The model under review builds one solid part; all positions refer to its coordinate system, in mm. Face numbers are marked on the shaded views. Coordinates: 2 decimals unless noted, no trailing zeros. Order: outer loops, then holes, each group sorted by start corner. A loop starts at its lowest first (then second) coordinate and runs counter-clockwise, first axis right, second up. Notation, with made-up numbers: M 8,-3 L 28,-3 A28 ccw 28,31 Z; hole C 29,-23.5 d9. An arc over 180 degrees is marked long. Write each question's results on one line, items separated by ' | '.
from build123d import *

# Parameters (mm, degrees)
SKETCH_R     = 2.5
SKETCH_R_2   = 1.6
PAD_DEPTH    = 3
SKETCH001_W  = 6.4
SKETCH001_H  = 103.817123
POCKET_DEPTH = 1


with BuildPart() as part:
    # Sketch → Pad (new body)
    with BuildSketch(Plane.XY):
        Polygon((0, 0), (38.400002, 0), (38.4, 61), (0, 61), align=None)
        with Locations((10, 46)):
            Circle(SKETCH_R, mode=Mode.SUBTRACT)
        with Locations((10, 26)):
            Circle(SKETCH_R, mode=Mode.SUBTRACT)
        with Locations((10, 6)):
            Circle(SKETCH_R, mode=Mode.SUBTRACT)
        with Locations((21.5, 54)):
            Circle(SKETCH_R_2, mode=Mode.SUBTRACT)
        with Locations((21.5, 7)):
            Circle(SKETCH_R_2, mode=Mode.SUBTRACT)
        with Locations((34.900002, 7)):
            Circle(SKETCH_R_2, mode=Mode.SUBTRACT)
        with Locations((34.900002, 54)):
            Circle(SKETCH_R_2, mode=Mode.SUBTRACT)
        with Locations((34.900002, 30.5)):
            Circle(SKETCH_R_2, mode=Mode.SUBTRACT)
        with Locations((21.5, 30.5)):
            Circle(SKETCH_R_2, mode=Mode.SUBTRACT)
    extrude(amount=PAD_DEPTH)

    # Sketch001 (on Face15 of Pad) → Pocket (cut)
    with BuildSketch(Plane.XY.offset(3)):
        with Locations((28.2, 19.77481)):
            Rectangle(SKETCH001_W, SKETCH001_H)
    extrude(amount=-POCKET_DEPTH, mode=Mode.SUBTRACT)


solid = part.part
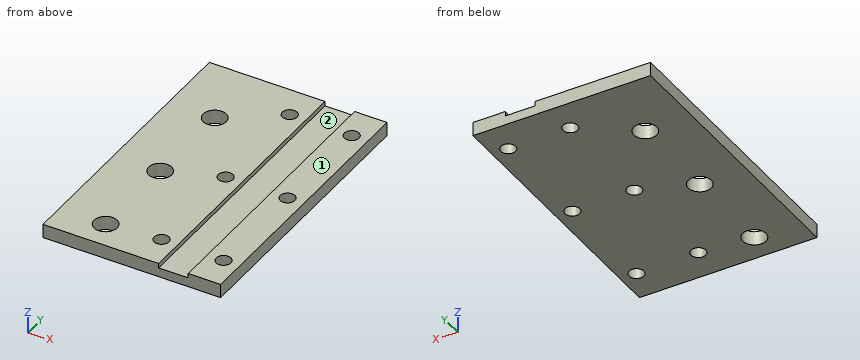
1) Take a section at C-C on z = 0.55. Count the separate pieces of the cut face and the enclosed holes in it, plus the area to 3 significant figures.
Solutions:
separate pieces: 1 | enclosed holes: 9 | area: 2,240 mm2
2) To check wall thickness, follow line 1 along Y through (x, z) = (21.5, 1.65); line 2 along Y through (x, z) = (10, 1.45); line 3 along X through (y, z) = (15, 2.25). State the ranges of each line that lie inside material, in increasing order.
Solutions:
line 1: 0 to 5.4, 8.6 to 28.9, 32.1 to 52.4, 55.6 to 61 | line 2: 0 to 3.5, 8.5 to 23.5, 28.5 to 43.5, 48.5 to 61 | line 3: 0 to 25, 31.4 to 38.4
3) For pin 1 (2 mm diameter, centred on x = 29, y = 27, fed in from +Z); pin 2 (4 mm diameter, centred on x = 10, y = 26, fed in from +Z); pin 3 (4 mm diameter, centred on x = 34.9, y = 54, fed in from +Z), all flat-tipped, find the tip position at first contact; note any pin that passes through.
Solutions:
pin 1: z = 2 | pin 2: through | pin 3: z = 3
4) Take a section at D-D on y = 19. State the section outline as (x, z) points.
Solutions:
outline: M 0,0 L 38.4,0 L 38.4,3 L 31.4,3 L 31.4,2 L 25,2 L 25,3 L 0,3 Z
5) Take a section at B-B on y = 30.5. State the section outline as (x, z) points.
Solutions:
outline: M 0,0 L 19.9,0 L 19.9,3 L 0,3 Z; M 23.1,0 L 33.3,0 L 33.3,3 L 31.4,3 L 31.4,2 L 25,2 L 25,3 L 23.1,3 Z; M 36.5,0 L 38.4,0 L 38.4,3 L 36.5,3 Z
6) The part is to be moulded in two halves that separate along X. For the marked faces 1 and 2, say which applies: pulls with the +X half, pulls with the -X half, needs draft (parallel to the pull), parting line crosses it, or undercut.
Solutions:
face 1: needs draft | face 2: undercut
7) Take a section at A-A on x = 10. State the section outline as (y, z) points, plus the area to 3 significant figures.
Solutions:
outline: M 0,0 L 3.5,0 L 3.5,3 L 0,3 Z; M 8.5,0 L 23.5,0 L 23.5,3 L 8.5,3 Z; M 28.5,0 L 43.5,0 L 43.5,3 L 28.5,3 Z; M 48.5,0 L 61,0 L 61,3 L 48.5,3 Z | area: 138 mm2
